Answer from the drawing. Dimensions are ordinates in mm from the lowest x, y and z of the part. A direction names the side the tool comes from. Give positions to 0.01 mm unless a question says otherwise; leave off trailing zeros. Order: outer loops, then holes, each group sorted by start corner. A loop starts at its lowest first (then second) coordinate and runs counter-clockwise, first axis right, second up. Notation, with made-up numbers: (69.25, 28.5) - (101.25, 28.5) arc R13 cw to (101.25, 44.5) - close; hole circle Ø11 at (-27.5, 58.5). An arc over 180 degrees is marked (long way). Answer in a Markdown table with one row per item.
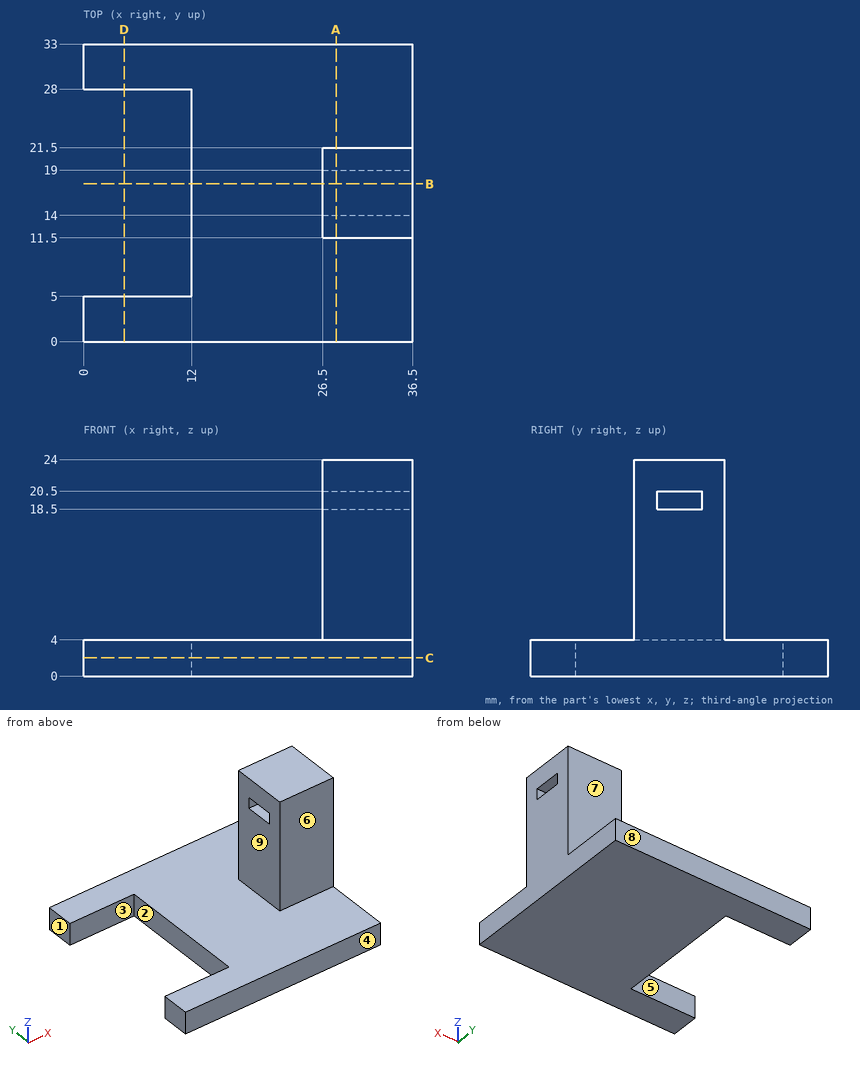
Item 1: Find section D-D on x = 4.5. Write down the section's boundary in (y, z).
Answer block:
| item | result |
|---|---|
| outline | (0, 0) - (5, 0) - (5, 4) - (0, 4) - close; (28, 0) - (33, 0) - (33, 4) - (28, 4) - close |
Item 2: Find section C-C on z = 2. Write down the section's boundary in (x, y).
Answer block:
| item | result |
|---|---|
| outline | (0, 0) - (36.5, 0) - (36.5, 33) - (0, 33) - (0, 28) - (12, 28) - (12, 5) - (0, 5) - close |
Item 3: Find section B-B on y = 17.5. Write down the section's boundary in (x, z).
Answer block:
| item | result |
|---|---|
| outline | (12, 0) - (36.5, 0) - (36.5, 18.5) - (26.5, 18.5) - (26.5, 4) - (12, 4) - close; (26.5, 20.5) - (36.5, 20.5) - (36.5, 24) - (26.5, 24) - close |
Item 4: Find section A-A on x = 28. Write down the section's boundary in (y, z).
Answer block:
| item | result |
|---|---|
| outline | (0, 0) - (33, 0) - (33, 4) - (21.5, 4) - (21.5, 24) - (11.5, 24) - (11.5, 4) - (0, 4) - close; hole (14, 18.5) - (19, 18.5) - (19, 20.5) - (14, 20.5) - close |
Item 5: Which of the six approach directions +Z, -Z, +X, -X, +Y, -Y give full straight-line access (tool end or side, diameter ignored) to the marked faces 5, 6, 7, 8 and 9?
Answer block:
| item | result |
|---|---|
| face 5 | +Z, -Z, -X |
| face 6 | +Z, +X, -X, -Y |
| face 7 | +Z, +X, -X, +Y |
| face 8 | +Z, -Z, +X, -X, +Y |
| face 9 | +Z, -X, +Y, -Y |
Item 6: Consider line 1 (Z direction, x = 31, y = 16.5); line 2 (Z direction, x = 12.5, y = 11); line 3 (Y direction, x = 35.5, z = 7). Determine where each line is inside the solid, lowest interval first.
Answer block:
| item | result |
|---|---|
| line 1 | 0 to 18.5, 20.5 to 24 |
| line 2 | 0 to 4 |
| line 3 | 11.5 to 21.5 |
Item 7: Each of these flat-tipped pins is pushed along its axis until it touches: P1, Ø3, axis at y = 18, z = 1, coming from the -X side; P2, Ø8, axis at y = 28.5, z = 21.5, coming from the -X side; P3, Ø5, axis at y = 15.5, z = 10, coming from the -X side; P4, Ø8, axis at x = 33.5, z = 10, coming from the -Y side. Where does it stop, or does it pass through?
Answer block:
| item | result |
|---|---|
| P1 | x = 12 |
| P2 | through |
| P3 | x = 26.5 |
| P4 | y = 11.5 |
Item 8: Determine the mould class of the marked faces 1, 2, 3 and 4 for opening direction Y: pulls with the +Y half, pulls with the -Y half, needs draft (parallel to the pull), parting line crosses it, or undercut.
Answer block:
| item | result |
|---|---|
| face 1 | needs draft |
| face 2 | undercut |
| face 3 | undercut |
| face 4 | pulls with the -Y half |
